from build123d import *

# Parameters (mm, degrees)
EXTRUDE_THIN1_DEPTH     = 40
CUT_EXTRUDE4_DEPTH      = 390.389022579
CUT_EXTRUDE4_DEPTH_BACK = 390.389022579
SKETCH2_W               = 80
SKETCH2_H               = 22


with BuildPart() as part:
    # Sketch1 → Extrude-Thin1 (new, symmetric)
    with BuildSketch(Plane.XY):
        Polygon((-15.1, 0), (0, 0), (7.44170041, 13.13891529), (14.88340082, 0), (22.325101231, 13.13891529), (29.766801641, 0), (37.208502051, 13.13891529), (44.650202461, 0), (52.091902871, 13.13891529), (59.533603282, 0), (66.975303692, 13.13891529), (74.417004102, 0), (81.858704512, 13.13891529), (89.300404922, 0), (96.742105333, 13.13891529), (104.183805743, 0), (111.625506153, 13.13891529), (119.067206563, 0), (126.508906973, 13.13891529), (133.950607384, 0), (141.392307794, 13.13891529), (148.834008204, 0), (156.275708614, 13.13891529), (163.717409024, 0), (171.159109435, 13.13891529), (178.600809845, 0), (186.042510255, 13.13891529), (193.484210665, 0), (200.925911075, 13.13891529), (208.367611485, 0), (215.809311896, 13.13891529), (223.251012306, 0), (230.692712716, 13.13891529), (238.134413126, 0), (245.576113536, 13.13891529), (253.017813947, 0), (260.459514357, 13.13891529), (267.901214767, 0), (275.342915177, 13.13891529), (282.784615587, 0), (290.226315998, 13.13891529), (297.668016408, 0), (305.109716818, 13.13891529), (312.551417228, 0), (319.993117638, 13.13891529), (327.434818049, 0), (334.876518459, 13.13891529), (342.318218869, 0), (349.759919279, 13.13891529), (357.201619689, 0), (364.6433201, 13.13891529), (372.08502051, 0), (387.08502051, 0), (387.08502051, 0.3), (372.259881967, 0.3), (364.6433201, 13.747647132), (357.201619689, 0.608731842), (349.759919279, 13.747647132), (342.318218869, 0.608731842), (334.876518459, 13.747647132), (327.434818049, 0.608731842), (319.993117638, 13.747647132), (312.551417228, 0.608731842), (305.109716818, 13.747647132), (297.668016408, 0.608731842), (290.226315998, 13.747647132), (282.784615587, 0.608731842), (275.342915177, 13.747647132), (267.901214767, 0.608731842), (260.459514357, 13.747647132), (253.017813947, 0.608731842), (245.576113536, 13.747647132), (238.134413126, 0.608731842), (230.692712716, 13.747647132), (223.251012306, 0.608731842), (215.809311896, 13.747647132), (208.367611485, 0.608731842), (200.925911075, 13.747647132), (193.484210665, 0.608731842), (186.042510255, 13.747647132), (178.600809845, 0.608731842), (171.159109435, 13.747647132), (163.717409024, 0.608731842), (156.275708614, 13.747647132), (148.834008204, 0.608731842), (141.392307794, 13.747647132), (133.950607384, 0.608731842), (126.508906973, 13.747647132), (119.067206563, 0.608731842), (111.625506153, 13.747647132), (104.183805743, 0.608731842), (96.742105333, 13.747647132), (89.300404922, 0.608731842), (81.858704512, 13.747647132), (74.417004102, 0.608731842), (66.975303692, 13.747647132), (59.533603282, 0.608731842), (52.091902871, 13.747647132), (44.650202461, 0.608731842), (37.208502051, 13.747647132), (29.766801641, 0.608731842), (22.325101231, 13.747647132), (14.88340082, 0.608731842), (7.44170041, 13.747647132), (-0.174861457, 0.3), (-15.1, 0.3), align=None)
    extrude(amount=EXTRUDE_THIN1_DEPTH, both=True)

    # Sketch2 → Cut-Extrude4 (cut, two sides: drawn at the far end of the back side and taken through both)
    with BuildSketch(Plane(origin=(0, 0, 0), x_dir=(1, 0, 0), z_dir=(0, 1, 0)).offset(-CUT_EXTRUDE4_DEPTH_BACK)):
        with Locations((347.08502051, -5)):
            Rectangle(SKETCH2_W, SKETCH2_H)
    extrude(amount=CUT_EXTRUDE4_DEPTH + CUT_EXTRUDE4_DEPTH_BACK, mode=Mode.SUBTRACT)


solid = part.part
For this review, take the finished solid that the model builds, in its own axes (mm). A direction names the side the tool comes from. Coordinates: 2 decimals unless noted, no trailing zeros. Write each loop counter-clockwise with the first axis right and the second up, starting at its lowest first coordinate (ties: lowest second). Pieces come first, ordered by that corner, then holes. Notation, with made-up numbers: (53.5, 55.5) -> (110.5, 55.5) arc R26 cw to (110.5, 70.5) -> close; hole circle Ø10 at (5.25, 29). An arc over 180 degrees is marked (long way). Write each question's results on one line, items separated by ' | '. Start each with the question number.
1) Wall thickness on L1, parallel to Y at x = 98.5, z = 7; L2, parallel to Y at x = 160.5, z = 14.5: over which ranges is each line inside the solid? List them lowest first. Write a range as [from, to].
2) The part is to be moulded in two halves that separate along X. For faces 4 (the face through (380, 0.3, 28)), 5 (the face through (227.024, 7.27, 0.56)), say which applies: +X half, -X half, draft (parallel to the pull), parting line (faces both ways), or undercut.
3) Consider section A-A (y = 5.5). Give the number of separate pieces and of enclosed holes in the cut face, plus the area to 3 significant figures.
4) Insertion check: pin 1 (4.5 mm diameter, centred on x = 378, z = -18.5, fed in from +Y); pin 2 (1.5 mm diameter, centred on y = 12.5, z = -26, fed in from +X); pin 3 (1 mm diameter, centred on x = 110.5, z = 15.5, fed in from -Y). Each pin has a flat end and moves straight along its axis. Give the tip position at first contact, or say it passes through.
5) Consider section B-B (x = 212.5). Write out the cut boundary in (y, z).
6) For faces 1 (the face through (316.324, 7.27, -22.762)), 2 (the face through (323.662, 6.661, -22.762)), 3 (the face through (380, 0.3, -23)), list the 3-axis set-ups (+Z, -Z, +X, -X, +Y, -Y) from which the entire face can be reached by the end or side of a thin tool; tool diameter is ignored.
Geometry says:
1) L1: [10.04, 10.64] | L2: [5.68, 6.29]
2) face 4: draft | face 5: undercut
3) separate pieces: 59 | enclosed holes: 0 | area: 1,310 mm^2
4) pin 1: y = 0.3 | pin 2: x = 365.77 | pin 3: y = 10.27
5) outline: (7.3, -40) -> (7.9, -40) -> (7.9, 40) -> (7.3, 40) -> close
6) face 1: +Z, -Z, +Y | face 2: +Z, -Z, -Y | face 3: +Z, -Z, +X, +Y
